Can you work these out from the model? Positions are in its coordinate system, mm. Face numbers are marked on the shaded views. A direction names the side the tool comes from. Give positions to 0.01 mm unless a question says otherwise; leave off trailing zeros. Loops run counter-clockwise (first coordinate to the right, second up) from the corner with the lowest first, then second, coordinate; pieces in that order, holes last. Notation, with made-up numbers: (68, -18) - (109, -18) arc R17 ccw to (109, 9) - close; hole circle Ø11 at (-34.5, -29.5). An arc over 180 degrees is marked (long way). Use a Markdown table: item, result. Add a question column.
```python
from build123d import *

# Parameters (mm, degrees)
F0_R     = 1
F1_DEPTH = 4
F2_START = 3
F2_DEPTH = 5


with BuildPart() as f1:
    # F0 (on Top) → F1 (new body)
    with BuildSketch(Plane.XY):
        Polygon((-2, 1.1547005384), (-2, -1.1547005384), (0, -2.3094010768), (2, -1.1547005384), (2, 1.1547005384), (0, 2.3094010768), align=None)
        Circle(F0_R, mode=Mode.SUBTRACT)
    extrude(amount=F1_DEPTH)

    # F0 (on Top) → F2 (join)
    with BuildSketch(Plane.XY.offset(F2_START)):
        Circle(F0_R)
    extrude(amount=F2_DEPTH)


solid = f1.part
```
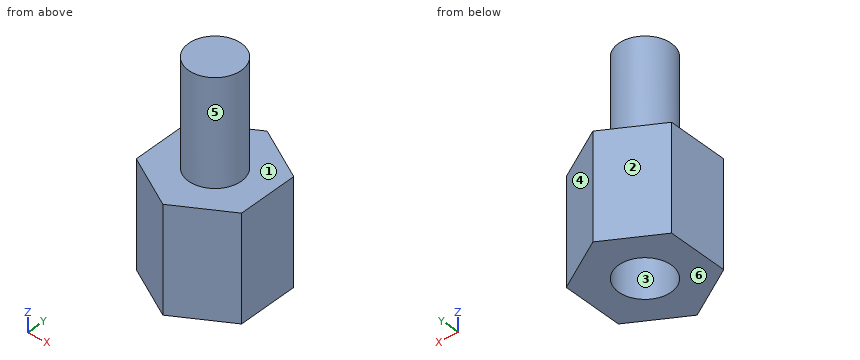
1. Suppose I cut it at B-B (z = 6.5). List the corners of the cut face in (x, y) for me, and give its area (3 significant figures).
2. Suppose I cut it at D-D (z = 3.5). List the corners of the cut face in (x, y) for me.
3. Will this pin go through, and if not, where does the flat tip stop? P1, Ø1.6, axis at x = 0, y = 0.5, coming from the -Z side.
4. Please list where these lines run through material, in increasing order: line 1 along Z through (x, y) = (0.6, -1.65); line 2 along Y through (x, z) = (0.75, 2); line 3 along Z through (x, y) = (0.15, -0.45). Write a range as [from, to].
5. Suppose I cut it at A-A (y = 0). List the corners of the cut face in (x, z) for me, and give its area (3 significant figures).
6. On a 3-axis mill with a long thin cutter (end or side, diameter ignored), from which of +Z, -Z, +X, -X, +Y, -Y can I reach the whole of each face in a straight line? I mean the marked faces 1 and 2. Say none if no direction works.
7. If we mould it in two halves opening along Y, with no side actions, what happens to the marked faces 3, 4, 5 and 6? For each: released by +Y, released by -Y, zero draft, split by the parting line, or undercut.
8. Suppose I cut it at C-C (x = -0.8). List the corners of the cut face in (y, z) for me.
Results below:
| question | item | result |
|---|---|---|
| 1 | outline | circle Ø2 at (0, 0) |
| 1 | area | 3.14 mm² |
| 2 | outline | (-2, -1.15) - (0, -2.31) - (2, -1.15) - (2, 1.15) - (0, 2.31) - (-2, 1.15) - close |
| 3 | P1 | z = 0 |
| 4 | line 1 | [0, 4] |
| 4 | line 2 | [-1.88, -0.66], [0.66, 1.88] |
| 4 | line 3 | [3, 8] |
| 5 | outline | (-2, 0) - (-1, 0) - (-1, 3) - (1, 3) - (1, 0) - (2, 0) - (2, 4) - (1, 4) - (1, 8) - (-1, 8) - (-1, 4) - (-2, 4) - close |
| 5 | area | 18.0 mm² |
| 6 | face 1 | +Z |
| 6 | face 2 | +Z, -Z, -X, +Y |
| 7 | face 3 | undercut |
| 7 | face 4 | released by +Y |
| 7 | face 5 | split by the parting line |
| 7 | face 6 | zero draft |
| 8 | outline | (-1.85, 0) - (-0.6, 0) - (-0.6, 3) - (0.6, 3) - (0.6, 0) - (1.85, 0) - (1.85, 4) - (0.6, 4) - (0.6, 8) - (-0.6, 8) - (-0.6, 4) - (-1.85, 4) - close |
